from build123d import *

# Parameters (mm, degrees)
F0_R     = 32.0745936063
F1_DEPTH = 101.854
F2_R     = 15.24
F3_DEPTH = 2.54
F4_DEPTH = 2.54
F5_W     = 22.9380205274
F5_H     = 43.4183962643
F6_DEPTH = 35.56
F7_DEPTH = 25.4


with BuildPart() as f1:
    # F0 (on Right) → F1 (new body)
    with BuildSketch(Plane.YZ):
        Circle(F0_R)
    extrude(amount=F1_DEPTH)

    # F2
    f2_edges = [f1.edges().sort_by_distance(p)[0] for p in [
        (101.854, -32.074594, 0),
        (50.927, 32.074594, 0),
        (0, -32.074594, 0),
    ]]
    fillet(f2_edges, radius=F2_R)

    # F3 (add): a face of the model
    f3_faces = [f1.faces().sort_by_distance(p)[0] for p in [
        (101.854, 0, 0),
    ]]
    extrude(f3_faces, amount=F3_DEPTH)

    # F4 (add): a face of the model
    f4_faces = [f1.faces().sort_by_distance(p)[0] for p in [
        (0, 0, 0),
    ]]
    extrude(f4_faces, amount=F4_DEPTH)

    # F5 (on Front) → F6 (join)
    with BuildSketch(Plane.XZ):
        with Locations((36.352340132, -0.5461424589)):
            Rectangle(F5_W, F5_H)
    extrude(amount=F6_DEPTH)

    # F7 (add): a face of the model
    f7_faces = [f1.faces().sort_by_distance(p)[0] for p in [
        (104.394, 0, 0),
    ]]
    extrude(f7_faces, amount=-F7_DEPTH)


solid = f1.part
The model under review builds one solid part; all positions refer to its coordinate system, in mm. A direction names the side the tool comes from. Give positions to 0.01 mm unless a question says otherwise; leave off trailing zeros. Loops run counter-clockwise (first coordinate to the right, second up) from the corner with the lowest first, then second, coordinate; pieces in that order, holes last. Notation, with made-up numbers: (2, 15) -> (45, 15) arc R17 ccw to (45, 25) -> close; hole circle Ø2 at (13.25, 74). An arc over 180 degrees is marked (long way). Answer as a JSON object with one key per item and string values. Group by question number.
Q1. Take a section at B-B (y = 0). Write out the cut boundary in (x, z).
Q2. Take a section at D-D (x = 32). Write out the cut boundary in (y, z), plus the area to 3 significant figures.
Q3. Take a section at A-A (z = 0). Write out the cut boundary in (x, y).
Q4. Wall thickness on line 1 along Z through (x, y) = (20, 1); line 2 along Z through (x, y) = (15, 24.5); line 3 along Y through (x, z) = (43, 16.5): over which ranges is each line inside the solid? List them lowest first.
Q5. Take a section at C-C (x = 59.5). Write out the cut boundary in (y, z).
Q6. Insertion check: pin 1 (6 mm diameter, centred on y = -27, z = 5, fed in from +X); pin 2 (5.5 mm diameter, centred on x = 39.5, y = -31.5, fed in from +Z); pin 3 (1.5 mm diameter, centred on x = 29, y = 9.5, fed in from +Z). Each pin has a flat end and moves straight along its axis. Give the tip position at first contact, or say it passes through.
Q7. Tool access review of faces 1 (the flat face through (24.883, -33, -1)), 2 (the cylindrical face through (103.106, 7.768, -14.935)), 3 (the flat face through (36, -29, -22.255)): name each direction out of +Z, -Z, +X, -X, +Y, -Y from which nothing blocks a thin tool from reaching the whole face with its end or side.
Answer below:
{
 "1": {"outline": "(-2.54, -16.83) -> (0, -16.83) arc R15.24 ccw to (15.24, -32.07) -> (86.61, -32.07) arc R15.24 ccw to (101.85, -16.83) -> (104.39, -16.83) -> (104.39, 16.83) -> (101.85, 16.83) arc R15.24 ccw to (86.61, 32.07) -> (15.24, 32.07) arc R15.24 ccw to (0, 16.83) -> (-2.54, 16.83) -> close"},
 "2": {"outline": "(-35.56, -22.26) -> (-23.1, -22.26) arc R32.07 ccw (long way) to (-24.1, 21.16) -> (-35.56, 21.16) -> close", "area": "3,500 mm2"},
 "3": {"outline": "(-2.54, -16.83) -> (0, -16.83) arc R15.24 ccw to (15.24, -32.07) -> (24.88, -32.07) -> (24.88, -35.56) -> (47.82, -35.56) -> (47.82, -32.07) -> (86.61, -32.07) arc R15.24 ccw to (101.85, -16.83) -> (104.39, -16.83) -> (104.39, 16.83) -> (101.85, 16.83) arc R15.24 ccw to (86.61, 32.07) -> (15.24, 32.07) arc R15.24 ccw to (0, 16.83) -> (-2.54, 16.83) -> close"},
 "4": {"line 1": "z = -32.06 to 32.06", "line 2": "z = -20.7 to 20.7", "line 3": "y = -35.56 to 27.51"},
 "5": {"outline": "circle Ø64.15 at (0, 0)"},
 "6": {"pin 1": "stops at x = 99.81", "pin 2": "stops at z = 21.16", "pin 3": "stops at z = 30.86"},
 "7": {"face 1": "-X, -Y", "face 2": "+X", "face 3": "-Z, +X, -X, -Y"}
}
